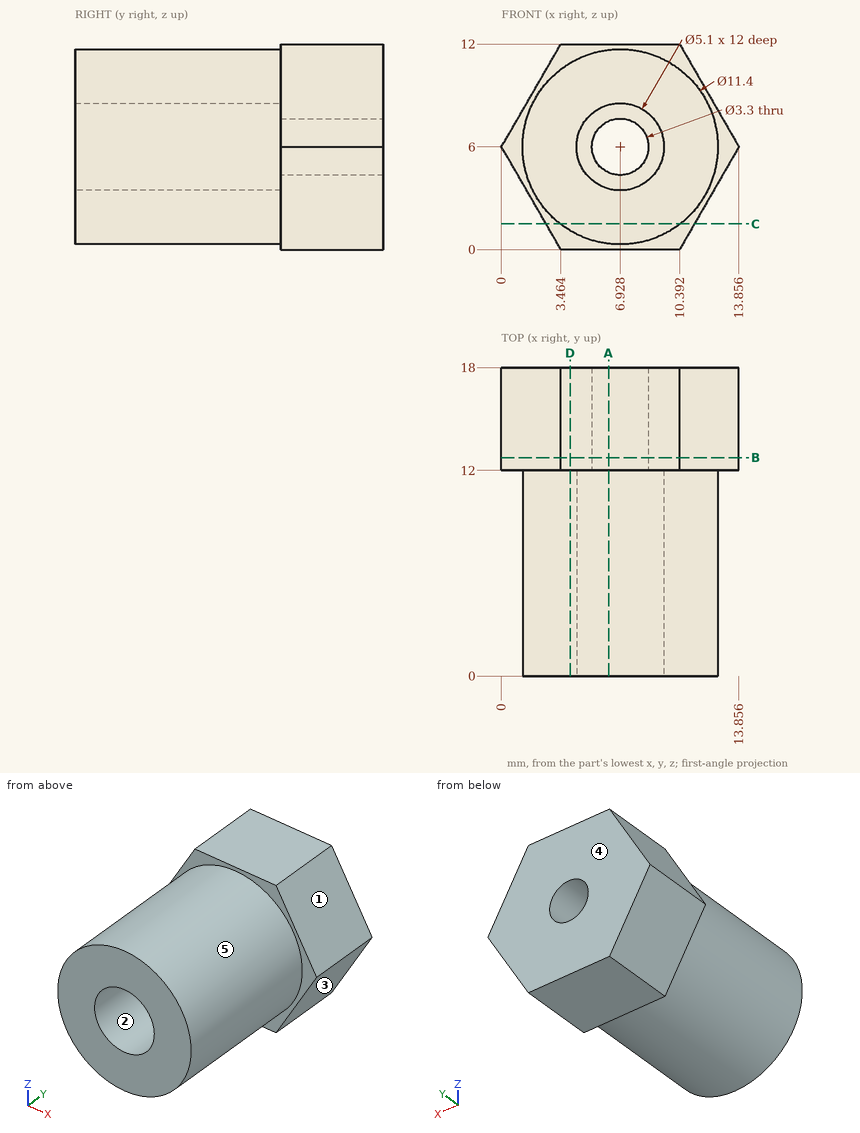
Geometry check sheet. Reference: drawing and pictorial views, mm from the part's lowest x, y, z. A direction names the side the tool comes from. Round coordinates to 2 decimals unless told otherwise and drop trailing zeros. Write each loop counter-clockwise with the first axis right and the second up, starting at its lowest first coordinate (ties: lowest second). Pieces come first, ordered by that corner, then holes. Notation, with made-up numbers: (62.25, -32) -> (95.25, -32) arc R27 ccw to (95.25, -10) -> close; hole circle Ø2 at (33, 64.5). An arc over 180 degrees is marked (long way). Answer as CSV lines item,"result". Start each with the question number.
1) Section check D-D on x = 4. Enter the section's corners in (y, z), and give its area (3 significant figures).
2) Section check C-C on z = 1.5. Enter the section's corners in (x, y), and give its area (3 significant figures).
3) Release check for a two-part mould opening along Z. For the marked faces 1, 2 and 3 record: pulls with the +Z half, pulls with the -Z half, needs draft (parallel to the pull), parting line crosses it, or undercut.
4) Material ranges on line 1 (X direction, y = 3, z = 6); line 2 (Y direction, x = 6.5, z = 4); line 3 (Z direction, x = 7.25, y = 5.5), recorded low to high. Write a range as from..to.
5) Go/stop test with flat-tipped pins: P1, Ø4, axis at x = 6.5, y = 5.5, coming from the -Z side; P2, Ø4.5, axis at x = 6.93, z = 6, coming from the +Y side; P3, Ø6, axis at x = 5, y = 2, coming from the +Z side. Record where each tip stops, or that it passes through.
6) Section check B-B on y = 12.75. Enter the section's corners in (x, z).
7) Tool access check on the marked faces 4 and 5. Record the directions out of +Z, -Z, +X, -X, +Y, -Y that give a thin tool (end or side, any length) a straight path to the whole face; none if there is none.
8) Section check A-A on x = 6.25. Enter the section's corners in (y, z), and give its area (3 significant figures).
Found:
1,outline,"(0, 1.11) -> (12, 1.11) -> (12, 0) -> (18, 0) -> (18, 12) -> (12, 12) -> (12, 10.89) -> (0, 10.89) -> close"
1,area,"189 mm^2"
2,outline,"(2.6, 12) -> (3.43, 12) -> (3.43, 0) -> (10.43, 0) -> (10.43, 12) -> (11.26, 12) -> (11.26, 18) -> (2.6, 18) -> close"
2,area,"136 mm^2"
3,face 1,"pulls with the +Z half"
3,face 2,"undercut"
3,face 3,"pulls with the -Z half"
4,line 1,"x = 1.23..4.38, 9.48..12.63"
4,line 2,"y = 12..18"
4,line 3,"z = 0.31..3.47, 8.53..11.69"
5,P1,"stops at z = 0.3"
5,P2,"stops at y = 18"
5,P3,"stops at z = 11.7"
6,outline,"(0, 6) -> (3.46, 0) -> (10.39, 0) -> (13.86, 6) -> (10.39, 12) -> (3.46, 12) -> close; hole circle Ø3.3 at (6.93, 6)"
7,face 4,"+Z, -Z, +X, -X, +Y"
7,face 5,"-Y"
8,outline,"(0, 0.34) -> (12, 0.34) -> (12, 0) -> (18, 0) -> (18, 4.5) -> (12, 4.5) -> (12, 3.54) -> (0, 3.54) -> close; (0, 8.46) -> (12, 8.46) -> (12, 7.5) -> (18, 7.5) -> (18, 12) -> (12, 12) -> (12, 11.66) -> (0, 11.66) -> close"
8,area,"131 mm^2"
